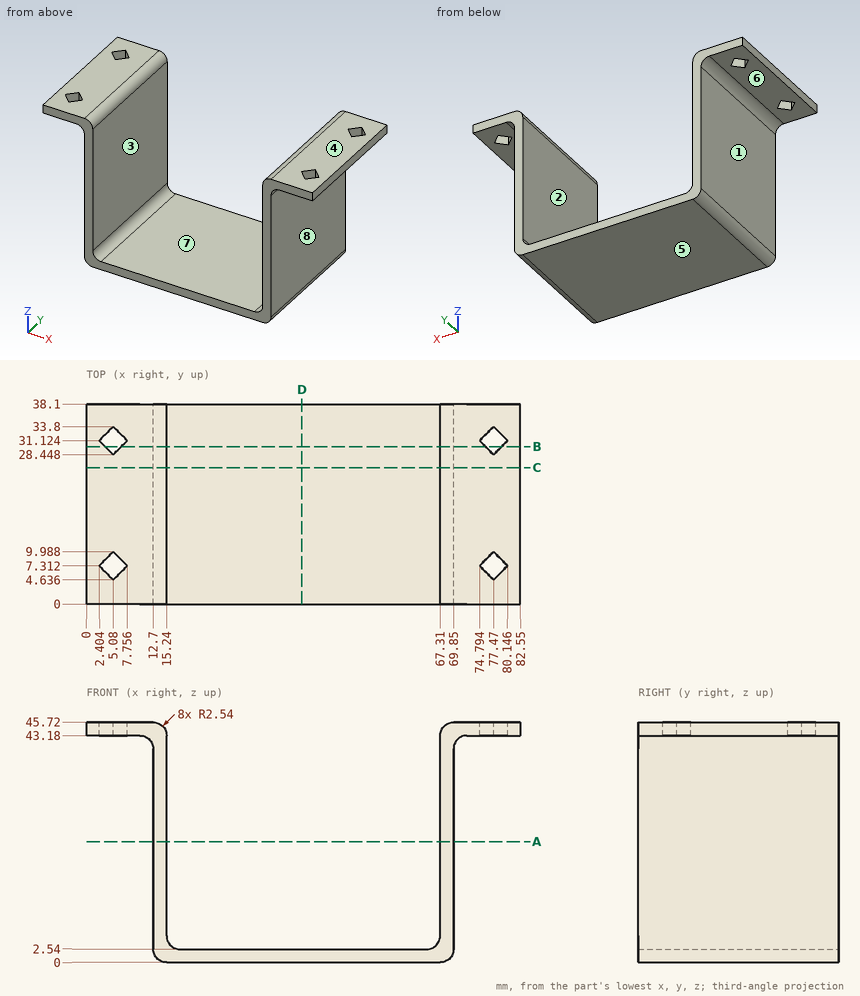
Geometry check sheet. Reference: drawing and pictorial views, mm from the part's lowest x, y, z. A direction names the side the tool comes from. Coordinates: 2 decimals unless noted, no trailing zeros. Order: outer loops, then holes, each group sorted by start corner. A loop starts at its lowest first (then second) coordinate and runs counter-clockwise, first axis right, second up. Notation, with made-up numbers: (-37, 86.5) -> (20, 86.5) arc R29 ccw to (20, 112.5) -> close; hole circle Ø7 at (56, 11.25). An arc over 180 degrees is marked (long way). Write item = value, one per line. Start each with the question number.
1) Go/stop test with flat-tipped pins: P1, Ø11.5, axis at y = 27, z = 29.5, coming from the -X side; P2, Ø3, axis at x = 79, y = 27.5, coming from the -Z side; P3, Ø8, axis at y = 23.5, z = 26, coming from the +X side. Record where each tip stops, or that it passes through.
2) Cross-section at D-D (x = 41). Enter the section's corners in (y, z).
3) Access from +Z, -Z, +X, -X, +Y, -Y to the whole of each face (thin tool, end or side, straight path). Record for the marked faces 5, 6, 7 and 8.
4) Cross-section at B-B (y = 30). Enter the section's corners in (x, z).
5) Material ranges on L1, parallel to X at y = 30, z = 21.5; L2, parallel to Z at x = 51, y = 11.5; L3, parallel to X at y = 36, z = 42 (1 decimal), recorded low to high.
6) Mould release check, pull along X, two halves, no side actions. Record for the marked faces 1, 2, 3 and 4: +X half, -X half, draft (parallel to the pull), parting line (faces both ways), or undercut.
7) Cross-section at C-C (y = 26). Enter the section's corners in (x, z), then the cut area to 3 significant figures.
8) Cross-section at A-A (z = 23). Enter the section's corners in (x, y).
Ans:
q1.P1 = 12.7
q1.P2 = 43.18
q1.P3 = 69.85
q2.outline = (0, 0) -> (38.1, 0) -> (38.1, 2.54) -> (0, 2.54) -> close
q3.face_5 = -Z, +X, -X, +Y, -Y
q3.face_6 = -Z, -X, +Y, -Y
q3.face_7 = +Z, +Y, -Y
q3.face_8 = -Z, +X, +Y, -Y
q4.outline = (0, 43.18) -> (3.53, 43.18) -> (3.53, 45.72) -> (0, 45.72) -> close; (6.63, 43.18) -> (10.16, 43.18) arc R2.54 cw to (12.7, 40.64) -> (12.7, 2.54) arc R2.54 ccw to (15.24, 0) -> (67.31, 0) arc R2.54 ccw to (69.85, 2.54) -> (69.85, 40.64) arc R2.54 cw to (72.39, 43.18) -> (75.92, 43.18) -> (75.92, 45.72) -> (69.85, 45.72) arc R2.54 ccw to (67.31, 43.18) -> (67.31, 5.08) arc R2.54 cw to (64.77, 2.54) -> (17.78, 2.54) arc R2.54 cw to (15.24, 5.08) -> (15.24, 43.18) arc R2.54 ccw to (12.7, 45.72) -> (6.63, 45.72) -> close; (79.02, 43.18) -> (82.55, 43.18) -> (82.55, 45.72) -> (79.02, 45.72) -> close
q5.L1 = 12.7 to 15.24, 67.31 to 69.85
q5.L2 = 0 to 2.54
q5.L3 = 12.3 to 15.2, 67.3 to 70.2
q6.face_1 = -X half
q6.face_2 = undercut
q6.face_3 = undercut
q6.face_4 = draft
q7.outline = (0, 43.18) -> (10.16, 43.18) arc R2.54 cw to (12.7, 40.64) -> (12.7, 2.54) arc R2.54 ccw to (15.24, 0) -> (67.31, 0) arc R2.54 ccw to (69.85, 2.54) -> (69.85, 40.64) arc R2.54 cw to (72.39, 43.18) -> (82.55, 43.18) -> (82.55, 45.72) -> (69.85, 45.72) arc R2.54 ccw to (67.31, 43.18) -> (67.31, 5.08) arc R2.54 cw to (64.77, 2.54) -> (17.78, 2.54) arc R2.54 cw to (15.24, 5.08) -> (15.24, 43.18) arc R2.54 ccw to (12.7, 45.72) -> (0, 45.72) -> close
q7.area = 429 mm²
q8.outline = (12.7, 0) -> (15.24, 0) -> (15.24, 38.1) -> (12.7, 38.1) -> close; (67.31, 0) -> (69.85, 0) -> (69.85, 38.1) -> (67.31, 38.1) -> close
